The listing builds one solid part. Answer for the finished solid, in the listing's coordinates (mm). Face numbers are marked on the shaded views. A direction names the side the tool comes from. Round coordinates to 2 decimals unless told otherwise and drop trailing zeros. Write each loop counter-clockwise with the first axis right and the second up, starting at its lowest first coordinate (ties: lowest second). Pieces come first, ordered by that corner, then holes. Notation, with made-up numbers: M -11.5,80.5 L 2.5,80.5 A26 ccw 2.5,104.5 Z; hole C -19,6 d6. An arc over 180 degrees is marked long. Answer as CSV lines item,"result". Start each with the question number.
from build123d import *

# Parameters (mm, degrees)
SKETCH1_W           = 15.8
SKETCH1_H           = 31.9
BOSS_EXTRUDE1_DEPTH = 2
SKETCH2_W           = 15.8
SKETCH2_H           = 31.9
SKETCH2_W_2         = 11.9
SKETCH2_H_2         = 22.6
BOSS_EXTRUDE3_DEPTH = 16.6
SKETCH3_R           = 1
CUT_EXTRUDE1_DEPTH  = 10
SKETCH4_W           = 4.5
SKETCH4_H           = 1.8
CUT_EXTRUDE2_DEPTH  = 38.762150362
SKETCH5_W           = 1.95
SKETCH5_H           = 31.9
CUT_EXTRUDE3_DEPTH  = 16.6
SKETCH6_W           = 4.65
SKETCH6_H           = 3
CUT_EXTRUDE4_DEPTH  = 10
BOSS_EXTRUDE4_DEPTH = 2.9


with BuildPart() as part:
    # Sketch1 → Boss-Extrude1 (new body)
    with BuildSketch(Plane(origin=(0, 0, 0), x_dir=(1, 0, 0), z_dir=(0, 1, 0))):
        Rectangle(SKETCH1_W, SKETCH1_H)
    extrude(amount=BOSS_EXTRUDE1_DEPTH)

    # Sketch2 → Boss-Extrude3 (add)
    with BuildSketch(Plane(origin=(0, 2, 0), x_dir=(1, 0, 0), z_dir=(0, 1, 0))):
        Rectangle(SKETCH2_W, SKETCH2_H)
        Rectangle(SKETCH2_W_2, SKETCH2_H_2, mode=Mode.SUBTRACT)
    extrude(amount=BOSS_EXTRUDE3_DEPTH)

    # Sketch3 → Cut-Extrude1 (cut)
    with BuildSketch(Plane(origin=(0, 18.6, 0), x_dir=(1, 0, 0), z_dir=(0, 1, 0))):
        with Locations(Location((0, 13.65, 0), (0, 0, 270))):
            Circle(SKETCH3_R)
        with Locations(Location((0, -13.65, 0), (0, 0, 90))):
            Circle(SKETCH3_R)
    extrude(amount=-CUT_EXTRUDE1_DEPTH, mode=Mode.SUBTRACT)

    # Sketch4 → Cut-Extrude2 (cut, through all)
    with BuildSketch(Plane.XY.offset(15.95)):
        with Locations((0, 16.7)):
            Rectangle(SKETCH4_W, SKETCH4_H)
    extrude(amount=-CUT_EXTRUDE2_DEPTH, mode=Mode.SUBTRACT)

    # Sketch5 → Cut-Extrude3 (cut)
    with BuildSketch(Plane(origin=(0, 18.6, 0), x_dir=(1, 0, 0), z_dir=(0, 1, 0))):
        with Locations((-6.925, 0)):
            Rectangle(SKETCH5_W, SKETCH5_H)
    extrude(amount=-CUT_EXTRUDE3_DEPTH, mode=Mode.SUBTRACT)

    # Sketch6 → Cut-Extrude4 (cut)
    with BuildSketch(Plane.ZY.offset(5.95)):
        with Locations((13.625, 8)):
            Rectangle(SKETCH6_W, SKETCH6_H)
    cut_extrude4 = extrude(amount=-CUT_EXTRUDE4_DEPTH, mode=Mode.SUBTRACT)

    # Sketch7 → Boss-Extrude4 (add)
    with BuildSketch(Plane.XZ):
        Polygon((7.9, 15.55), (-7.9, 15.55), (-7.9, 12.55), (5.9, 12.55), (5.9, -12.55), (-7.9, -12.55), (-7.9, -15.55), (7.9, -15.55), align=None)
    extrude(amount=BOSS_EXTRUDE4_DEPTH)

    # Mirror1: Cut-Extrude4 across plane
    add(cut_extrude4.mirror(Plane.XY), mode=Mode.SUBTRACT)


solid = part.part
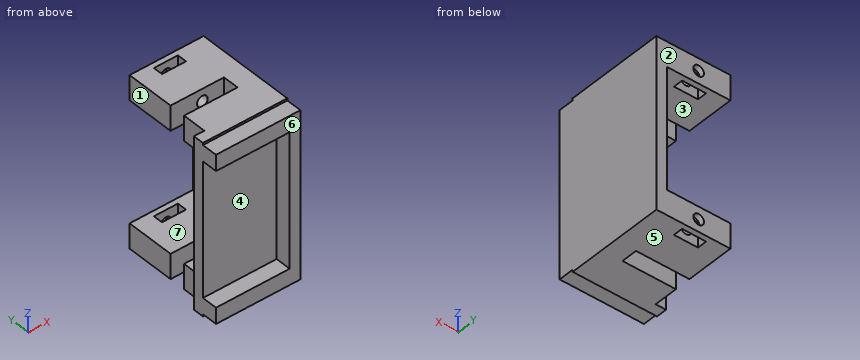
Q1. Find section D-D (y = 12.5). Determine the outline of the cut face in (x, z).
Q2. For the marked faces 1, 2 and 3, determine the directions among +Z, -Z, +X, -X, +Y, -Y from which every point of the face is accessible in a straight line to the end or side of a thin tool.
Q3. Each of these flat-tipped pins is pushed along its axis until it touches: P1, Ø2, axis at x = -5, z = 2, coming from the -Y side; P2, Ø3, axis at x = -5.5, z = -9.5, coming from the +Y side; P3, Ø1.4, axis at x = 2, y = -2, coming from the -Z side. Where does it stop, or does it pass through?
Q4. Straight lines are drawn through the part: L1, parallel to Z at x = 3.5, y = 11.75; L2, parallel to X at y = 18.4, z = -13.65; L3, parallel to X at y = 5.5, z = -13. For each, find the intervals that lie inside material, in ascending order.
Q5. Find section B-B (z = 13.65). Determine the outline of the cut face in (x, y).
Q6. Find section C-C (x = -4). Determine the outline of the cut face in (y, z).
Q7. Find section A-A (y = 16.5). Determine the outline of the cut face in (x, z), plus the area to 3 significant figures.
Q8. The mould has two halves that part along Z. Classify the marked faces 4, 5, 6 and 7: +Z half, -Z half, draft (parallel to the pull), parting line (faces both ways), or undercut.
Reported:
1,outline,"M -5.95,-15.95 L 7.9,-15.95 L 7.9,15.95 L -5.95,15.95 L -5.95,11.3 L 5.95,11.3 L 5.95,-11.3 L -5.95,-11.3 Z; hole C 0,-13.65 d2; hole C 0,13.65 d2"
2,face 1,"+Z, -Z, -X, +Y"
2,face 2,"+Z, -Z, +X, -X, +Y"
2,face 3,"-X, +Y"
3,P1,"stops at y = 0"
3,P2,"stops at y = 2"
3,P3,"stops at z = -15.55"
4,L1,"z = -15.95 to -11.3, 11.3 to 15.95"
4,L2,"x = -5.95 to -1, 1 to 7.9"
4,L3,"x = -5.95 to 7.9"
5,outline,"M -7.9,-2.9 L 7.9,-2.9 L 7.9,18.6 L 1,18.6 L 1,17.6 L 2.25,17.6 L 2.25,15.8 L 1,15.8 L 1,9.5 L 4.05,9.5 L 4.05,6.5 L -5.95,6.5 L -5.95,2 L -7.9,2 Z; M -5.95,9.5 L -1,9.5 L -1,15.8 L -2.25,15.8 L -2.25,17.6 L -1,17.6 L -1,18.6 L -5.95,18.6 Z"
6,outline,"M -2.9,-15.55 L 0,-15.55 L 0,-15.95 L 6.5,-15.95 L 6.5,-11.3 L 2,-11.3 L 2,11.3 L 6.5,11.3 L 6.5,15.95 L 0,15.95 L 0,15.55 L -2.9,15.55 L -2.9,12.55 L 0,12.55 L 0,-12.55 L -2.9,-12.55 Z; M 9.5,-15.95 L 18.6,-15.95 L 18.6,-11.3 L 9.5,-11.3 Z; M 9.5,11.3 L 18.6,11.3 L 18.6,15.95 L 9.5,15.95 Z"
7,outline,"M -5.95,-15.95 L -2.25,-15.95 L -2.25,-11.3 L -5.95,-11.3 Z; M -5.95,11.3 L -2.25,11.3 L -2.25,15.95 L -5.95,15.95 Z; M 2.25,-15.95 L 7.9,-15.95 L 7.9,15.95 L 2.25,15.95 L 2.25,11.3 L 5.95,11.3 L 5.95,-11.3 L 2.25,-11.3 Z"
7,area,"131 mm2"
8,face 4,"undercut"
8,face 5,"-Z half"
8,face 6,"draft"
8,face 7,"undercut"
